Build history of the part. All positions in model axes, mm. Face numbers are marked on the shaded views. A direction names the side the tool comes from. Give positions to 0.01 mm unless a question says otherwise; leave off trailing zeros. Loops run counter-clockwise (first coordinate to the right, second up) from the corner with the lowest first, then second, coordinate; pieces in that order, holes last.
1) Band-saw the part on B-B on x = 0. List the corners of the cut face in (y, z).
2) Band-saw the part on D-D on y = 12.75. List the corners of the cut face in (x, z).
3) Two-plate mould, pull along X, no slides. Class the marked faces 1, 2 and 3: +X half, -X half, draft (parallel to the pull), parting line (faces both ways), or undercut.
4) Band-saw the part on A-A on z = 0. List the corners of the cut face in (x, y), then the cut area to 3 significant figures.
5) 3-axis set-ups, long thin cutter, end or side, ignore diameter. For the marked faces 4 and 5: which of +Z, -Z, +X, -X, +Y, -Y reach the whole face in a straight line?
6) Flat gauge pins, fed straight in: P1, Ø5, axis at x = -5, y = 4.5, coming from the +Z side; P2, Ø5, axis at y = 2.5, z = -7, coming from the -X side; P3, Ø5, axis at y = 12.5, z = -7.5, coming from the +X side. Where does each tip first touch, or does it go through?
7) Wall check: line 1 (Y direction, x = 1.75, z = -7); line 2 (X direction, y = 4.25, z = 1.5); line 3 (Z direction, x = -1, y = 3.25). Give the ranges that are in metal, low to high.
8) Band-saw the part on C-C on y = 2.5. List the corners of the cut face in (x, z).
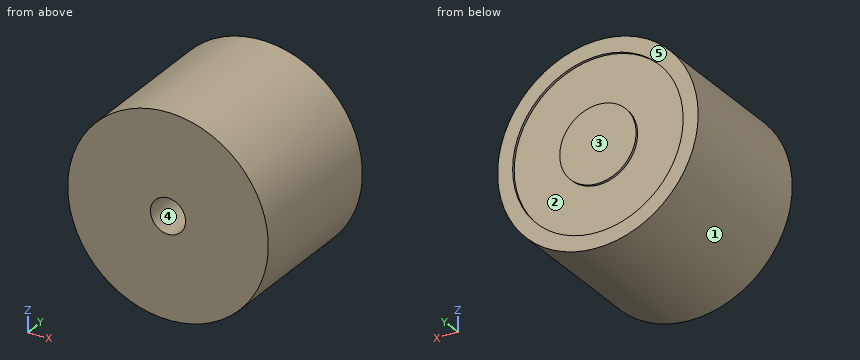
Autodesk Inventor part; units mm, degrees
ref_plane "YZ Plane" through (0, 0, 0) normal (1, 0, 0) x (0, 1, 0)
ref_plane "XZ Plane" through (0, 0, 0) normal (0, 1, 0) x (-1, 0, 0)
ref_plane "XY Plane" through (0, 0, 0) normal (0, 0, 1) x (1, 0, 0)
sketch "Sketch1" plane through (0, 0, 0) normal (0, 1, 0) x (-1, 0, 0)
  circle A0 centre (0, 0) radius 10.0076
  dimension "d0" = 20.0152
extrude "Extrusion1" add sketch "Sketch1" along normal blind 15.0876
sketch "Sketch2" plane through (0, 15.0876, 0) normal (0, 1, 0) x (1, 0, 0)
  circle A0 centre (0, 0) radius 3.81
  circle A1 centre (0, 0) radius 8.509
  dimension "d3" = 7.62
  dimension "d4" = 17.018
extrude "Extrusion2" cut sketch "Sketch2" against normal blind 0.254
sketch "Sketch3" plane through (0, 0, 0) normal (0, -1, 0) x (1, 0, 0)
  circle A0 centre (0, 0) radius 1.75
  dimension "d7" = 3.5
extrude "Extrusion3" cut sketch "Sketch3" against normal blind 5.08
thread "Thread1"
properties part number "electromagnet" material "Stainless Steel"
Findings below:
1. outline: (0, -10.01) - (15.09, -10.01) - (15.09, -8.51) - (14.83, -8.51) - (14.83, -3.81) - (15.09, -3.81) - (15.09, 3.81) - (14.83, 3.81) - (14.83, 8.51) - (15.09, 8.51) - (15.09, 10.01) - (0, 10.01) - (0, 1.75) - (5.08, 1.75) - (5.08, -1.75) - (0, -1.75) - close
2. outline: circle Ø20.02 at (0, 0)
3. face 1: parting line
3. face 2: undercut
3. face 3: draft
4. outline: (-10.01, 0) - (-1.75, 0) - (-1.75, 5.08) - (1.75, 5.08) - (1.75, 0) - (10.01, 0) - (10.01, 15.09) - (8.51, 15.09) - (8.51, 14.83) - (3.81, 14.83) - (3.81, 15.09) - (-3.81, 15.09) - (-3.81, 14.83) - (-8.51, 14.83) - (-8.51, 15.09) - (-10.01, 15.09) - close
4. area: 282 mm2
5. face 4: -Y
5. face 5: +Z, -Z, +X, -X, +Y
6. P1: stops at z = 9.69
6. P2: stops at x = -8.94
6. P3: stops at x = 8.67
7. line 1: y = 0 to 14.83
7. line 2: x = -9.89 to -0.9, 0.9 to 9.89
7. line 3: z = -9.96 to -1.44, 1.44 to 9.96
8. outline: circle Ø20.02 at (0, 0); hole circle Ø3.5 at (0, 0)
